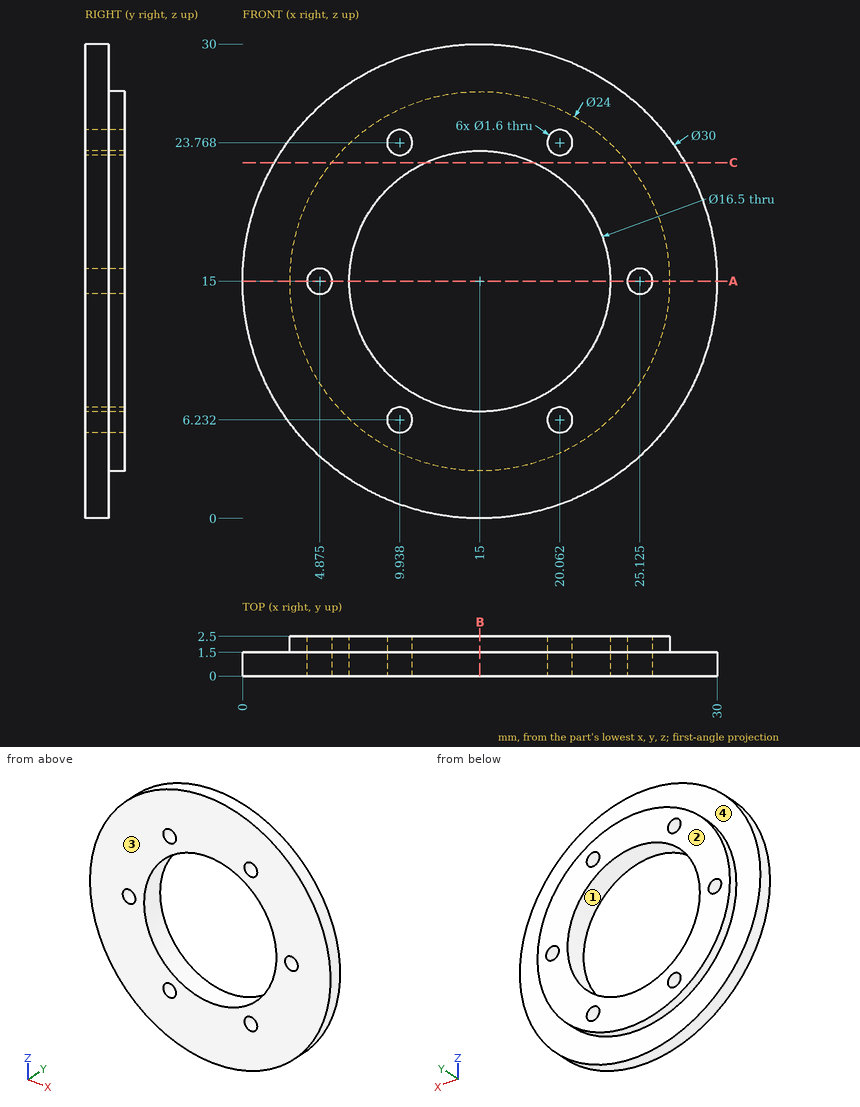
Study the drawing (mm; zero at the part's minimum x, y, z) and answer. A direction names the side the tool comes from. Give positions to 0.01 mm unless a question says otherwise; leave off trailing zeros. Write each loop counter-clockwise with the first axis right and the second up, starting at its lowest first coordinate (ties: lowest second). Pieces come first, ordered by that corner, then holes. Notation, with made-up numbers: (42.5, 74.25) -> (88.5, 74.25) arc R22 ccw to (88.5, 85.25) -> close; hole circle Ø7 at (-20.75, 73). An arc over 180 degrees is marked (long way). Write item = value, one per line. Start each with the question number.
1) The part is cut by section B-B, the plane x = 15. Determine the outline of the cut face in (y, z).
2) The part is cut by section A-A, the plane z = 15. Count the separate pieces of the cut face and the enclosed holes in it.
3) This flat-tipped pin is pushed along its axis until it touches: pin 1 (2 mm diameter, centred on x = 20.06, z = 23.77, fed in from -Y). Where does it stop, or does it pass through?
4) Straight lines are drawn through the part: line 1 along Z through (x, y) = (15, 1.1); line 2 along Z through (x, y) = (10.5, 0.7) (1 decimal); line 3 along X through (y, z) = (0.75, 6.5) (1 decimal). For each, find the intervals that lie inside material, in ascending order.
5) Which of the six approach directions +Z, -Z, +X, -X, +Y, -Y give full straight-line access (tool end or side, diameter ignored) to the marked faces 3 and 4?
6) The part is cut by section C-C, the plane z = 22.5. Determine the outline of the cut face in (x, y).
7) Determine the mould class of the marked faces 1 and 2 for opening direction Z: +Z half, -Z half, draft (parallel to the pull), parting line (faces both ways), or undercut.
Solutions:
q1.outline = (0, 0) -> (1.5, 0) -> (1.5, 3) -> (2.5, 3) -> (2.5, 6.75) -> (0, 6.75) -> close; (0, 23.25) -> (2.5, 23.25) -> (2.5, 27) -> (1.5, 27) -> (1.5, 30) -> (0, 30) -> close
q2.separate_pieces = 4
q2.enclosed_holes = 0
q3.pin_1 = 0
q4.line_1 = 0 to 6.75, 23.25 to 30
q4.line_2 = 0.7 to 5.7, 6.8 to 8.1, 21.9 to 23.2, 24.3 to 29.3
q4.line_3 = 2.6 to 9.2, 10.7 to 19.3, 20.8 to 27.4
q5.face_3 = +Z, -Z, +X, -X, -Y
q5.face_4 = +Y
q6.outline = (2.01, 0) -> (11.56, 0) -> (11.56, 2.5) -> (5.63, 2.5) -> (5.63, 1.5) -> (2.01, 1.5) -> close; (18.44, 0) -> (27.99, 0) -> (27.99, 1.5) -> (24.37, 1.5) -> (24.37, 2.5) -> (18.44, 2.5) -> close
q7.face_1 = undercut
q7.face_2 = draft
